Here's how the part is built. I have some questions about the finished solid (model axes, mm). A direction names the side the tool comes from. Coordinates: 2 decimals unless noted, no trailing zeros. Write each loop counter-clockwise with the first axis right and the second up, starting at its lowest first coordinate (ties: lowest second). Pieces come first, ordered by that corner, then holes. Notation, with made-up numbers: (12.5, 9.5) -> (63.5, 9.5) arc R32 ccw to (63.5, 46.5) -> close; hole circle Ø5 at (64, -0.75). An arc over 180 degrees is marked (long way). Use CSV: the item, a comma, the result in double quotes. Start each with the question number.
```python
from build123d import *

# Parameters (mm, degrees)
SKETCH1_W           = 120
SKETCH1_H           = 100
BOSS_EXTRUDE1_DEPTH = 40
SKETCH2_W           = 112
SKETCH2_H           = 92
CUT_EXTRUDE1_DEPTH  = 36
SKETCH3_W           = 28
SKETCH3_H           = 70
BOSS_EXTRUDE3_DEPTH = 8
SKETCH6_W           = 24.21
SKETCH6_H           = 8
CUT_EXTRUDE4_DEPTH  = 66
CUT_EXTRUDE6_DEPTH  = 66


with BuildPart() as part:
    # Sketch1 → Boss-Extrude1 (new body)
    with BuildSketch(Plane(origin=(0, 0, 0), x_dir=(1, 0, 0), z_dir=(0, 1, 0))):
        with Locations((-10.571222942, 10.082692781)):
            Rectangle(SKETCH1_W, SKETCH1_H)
    extrude(amount=BOSS_EXTRUDE1_DEPTH)

    # Sketch2 → Cut-Extrude1 (cut)
    with BuildSketch(Plane(origin=(0, 40, 0), x_dir=(1, 0, 0), z_dir=(0, 1, 0))):
        with Locations((-10.571222942, 10.082692781)):
            Rectangle(SKETCH2_W, SKETCH2_H)
    extrude(amount=-CUT_EXTRUDE1_DEPTH, mode=Mode.SUBTRACT)

    # Sketch3 → Boss-Extrude3 (add)
    with BuildSketch(Plane(origin=(0, 4, 0), x_dir=(1, 0, 0), z_dir=(0, 1, 0))):
        with Locations((-42.571222942, 25.082692781)):
            Rectangle(SKETCH3_W, SKETCH3_H)
    extrude(amount=BOSS_EXTRUDE3_DEPTH)

    # Sketch6 → Cut-Extrude4 (cut)
    with BuildSketch(Plane.XY.offset(9.917307219)):
        with Locations((-42.569304131, 8)):
            Rectangle(SKETCH6_W, SKETCH6_H)
    extrude(amount=-CUT_EXTRUDE4_DEPTH, mode=Mode.SUBTRACT)

    # Sketch7 → Cut-Extrude6 (cut)
    with BuildSketch(Plane.XY.offset(-56.082692781)):
        Polygon((-54.674304131, 12), (-50.474304131, 12), (-50.474304131, 6.53), (-47.074304131, 6.53), (-47.074304131, 12), (-38.074304131, 12), (-38.074304131, 6.53), (-34.664304131, 6.53), (-34.664304131, 12), (-30.464304131, 12), (-30.464304131, 6.53), (-30.464304131, 4), (-54.674304131, 4), (-54.674304131, 6.53), align=None)
    extrude(amount=-CUT_EXTRUDE6_DEPTH, mode=Mode.SUBTRACT)


solid = part.part
```
Item 1: I want a section at B-B on x = 32. Please give me the cut outline in (y, z).
Item 2: I'm going to push a flat-ended pin straight in: pin 1 (0.6 mm diameter, centred on x = -30, z = -20, fed in from +Y). Where does the tip first touch, or does it pass through?
Item 3: If I drill on line 1 along Z through (x, y) = (12, 6); line 2 along X through (y, z) = (11, 2.5); line 3 along X through (y, z) = (17, 20.5), over which ranges is the centre line in solid material (lowest first)?
Item 4: I want a section at C-C on y = 32.5. Please give me the cut outline in (x, z).
Item 5: I want a section at D-D on z = -50. Please give me the cut outline in (x, y).
Item 6: I want a section at A-A on y = 8.5. Please give me the cut outline in (x, z).
Item 7: Thinking about a two-plate mould opening in Z: for faces 4 (the flat face through (-11, 20, -60.083)), 5 (the flat face through (-28.571, 8, -23)), 6 (the flat face through (-33, 12, -58)), 7 (the flat face through (-66.571, 22, -9)), which applies, +Z half, -Z half, draft (parallel to the pull), parting line (faces both ways), or undercut?
Item 8: Which directions (+Z, -Z, +X, -X, +Y, -Y) give clear straight access to the entire face, cutting with the end or side of a thin tool? Please do faces 1 (the flat face through (-43, 12, -58)), 2 (the flat face through (-11, 22, 35.917)), 3 (the flat face through (-11, 0, -11)).
Geometry says:
1,outline,"(0, -60.08) -> (40, -60.08) -> (40, -56.08) -> (4, -56.08) -> (4, 35.92) -> (40, 35.92) -> (40, 39.92) -> (0, 39.92) -> close"
2,pin 1,"y = 12"
3,line 1,"-60.08 to -56.08, 35.92 to 39.92"
3,line 2,"-70.57 to -66.57, -56.57 to -54.67, -30.46 to -28.57, 45.43 to 49.43"
3,line 3,"-70.57 to -66.57, 45.43 to 49.43"
4,outline,"(-70.57, -60.08) -> (49.43, -60.08) -> (49.43, 39.92) -> (-70.57, 39.92) -> close; hole (-66.57, -56.08) -> (45.43, -56.08) -> (45.43, 35.92) -> (-66.57, 35.92) -> close"
5,outline,"(-70.57, 0) -> (49.43, 0) -> (49.43, 40) -> (45.43, 40) -> (45.43, 4) -> (-28.57, 4) -> (-28.57, 12) -> (-30.46, 12) -> (-30.46, 4) -> (-54.67, 4) -> (-54.67, 12) -> (-56.57, 12) -> (-56.57, 4) -> (-66.57, 4) -> (-66.57, 40) -> (-70.57, 40) -> close"
6,outline,"(-70.57, -60.08) -> (-54.67, -60.08) -> (-54.67, 9.92) -> (-56.57, 9.92) -> (-56.57, -56.08) -> (-66.57, -56.08) -> (-66.57, 35.92) -> (45.43, 35.92) -> (45.43, -56.08) -> (-28.57, -56.08) -> (-28.57, 9.92) -> (-30.46, 9.92) -> (-30.46, -60.08) -> (49.43, -60.08) -> (49.43, 39.92) -> (-70.57, 39.92) -> close; (-50.47, -60.08) -> (-47.07, -60.08) -> (-47.07, -56.08) -> (-50.47, -56.08) -> close; (-38.07, -60.08) -> (-34.66, -60.08) -> (-34.66, -56.08) -> (-38.07, -56.08) -> close"
7,face 4,"-Z half"
7,face 5,"undercut"
7,face 6,"draft"
7,face 7,"undercut"
8,face 1,"-Z"
8,face 2,"+Y"
8,face 3,"+Z, -Z, +X, -X, -Y"
